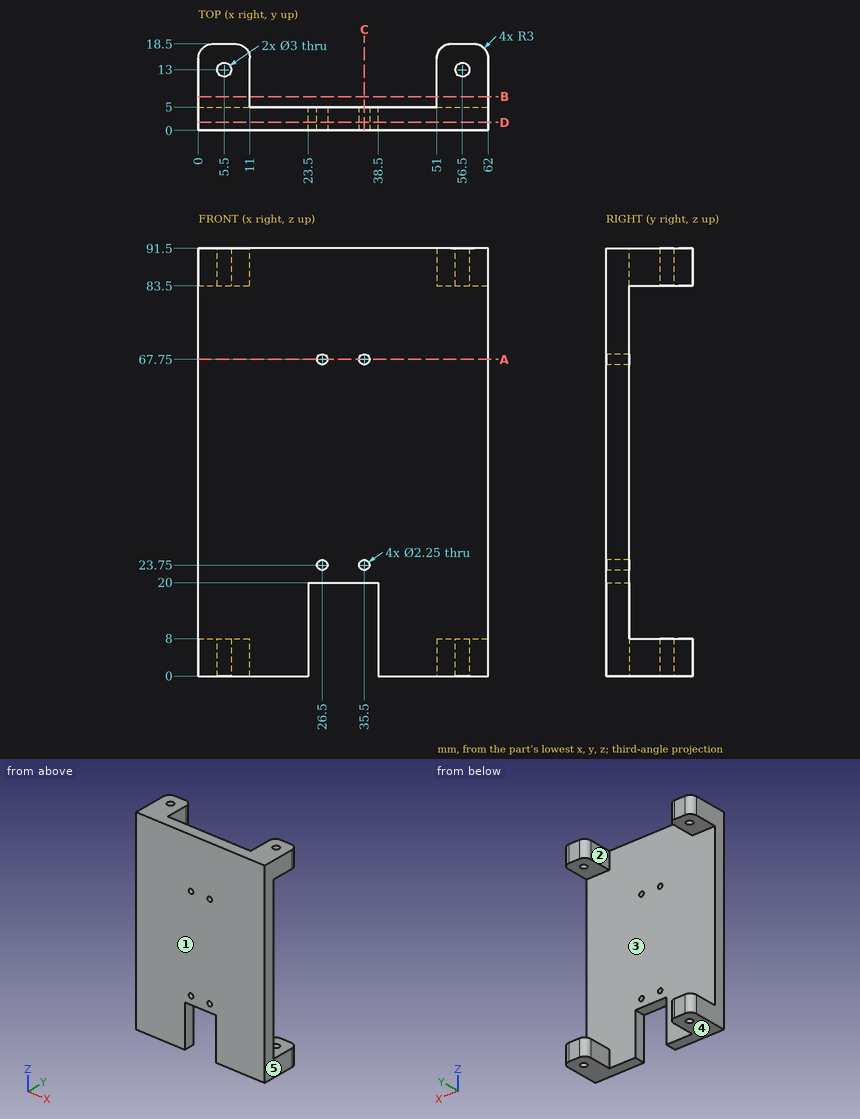
Here's the drawing with two shaded views (mm, measured from the low corner). I have some questions. A direction names the side the tool comes from. Give positions to 0.01 mm unless a question says otherwise; leave off trailing zeros. Write each loop counter-clockwise with the first axis right and the second up, starting at its lowest first coordinate (ties: lowest second). Pieces come first, ordered by that corner, then holes. Notation, with made-up numbers: (-25, -8) -> (-1, -8) arc R29 ccw to (-1, 17) -> close; hole circle Ø7 at (-17.75, 47.25). An arc over 180 degrees is marked (long way). Answer as a JSON object with one key per item and string values. Group by question number.
Item 1: Suppose I cut it at C-C (x = 35.5). Please give me the cut outline in (y, z) (3 decimals), plus the area to 3 significant figures.
Item 2: Suppose I cut it at D-D (y = 1.75). Please give me the cut outline in (x, z) (3 decimals).
Item 3: Suppose I cut it at B-B (y = 7.25). Please give me the cut outline in (x, z).
Item 4: We'd pull the mould along Z, two halves only. Please class the marked faces 3, 4 and 5: +Z half, -Z half, draft (parallel to the pull), parting line (faces both ways), or undercut.
Item 5: I'm going to push flat-ended pins straight in: P1, Ø2.5, axis at x = 5.5, y = 13, coming from the +Z side; P2, Ø3, axis at x = 35.5, z = 23.75, coming from the -Y side; P3, Ø1.5, axis at x = 29.5, y = 2, coming from the -Z side. Where does each tip first touch, or does it pass through?
Item 6: Please list where these lines run through material, in increasing order: line 1 (X direction, y = 3, z = 67.75) (3 decimals); line 2 (Z direction, x = 8, y = 8.25); line 3 (X direction, y = 4.5, z = 14.5). Write a range as [from, to].
Item 7: For the marked faces 1 and 2, which set-ups out of +Z, -Z, +X, -X, +Y, -Y let a thin tool reach every point of the face, with its end or its side?
Item 8: Suppose I cut it at A-A (z = 67.75). Please give me the cut outline in (x, y) (3 decimals).
Findings:
{
 "1": {"outline": "(0, 20) -> (5, 20) -> (5, 22.625) -> (0, 22.625) -> close; (0, 24.875) -> (5, 24.875) -> (5, 66.625) -> (0, 66.625) -> close; (0, 68.875) -> (5, 68.875) -> (5, 91.5) -> (0, 91.5) -> close", "area": "335 mm²"},
 "2": {"outline": "(0, 0) -> (23.5, 0) -> (23.5, 20) -> (38.5, 20) -> (38.5, 0) -> (62, 0) -> (62, 91.5) -> (0, 91.5) -> close; hole circle Ø2.25 at (26.5, 23.75); hole circle Ø2.25 at (26.5, 67.75); hole circle Ø2.25 at (35.5, 23.75); hole circle Ø2.25 at (35.5, 67.75)"},
 "3": {"outline": "(0, 0) -> (11, 0) -> (11, 8) -> (0, 8) -> close; (0, 83.5) -> (11, 83.5) -> (11, 91.5) -> (0, 91.5) -> close; (51, 0) -> (62, 0) -> (62, 8) -> (51, 8) -> close; (51, 83.5) -> (62, 83.5) -> (62, 91.5) -> (51, 91.5) -> close"},
 "4": {"face 3": "undercut", "face 4": "-Z half", "face 5": "draft"},
 "5": {"P1": "passes through", "P2": "stops at y = 0", "P3": "stops at z = 20"},
 "6": {"line 1": "x = [0, 25.375], [27.625, 34.375], [36.625, 62]", "line 2": "z = [0, 8], [83.5, 91.5]", "line 3": "x = [0, 23.5], [38.5, 62]"},
 "7": {"face 1": "+Z, -Z, +X, -X, -Y", "face 2": "+Z, -Z, +Y"},
 "8": {"outline": "(0, 0) -> (25.375, 0) -> (25.375, 5) -> (0, 5) -> close; (27.625, 0) -> (34.375, 0) -> (34.375, 5) -> (27.625, 5) -> close; (36.625, 0) -> (62, 0) -> (62, 5) -> (36.625, 5) -> close"}
}
